Check sheet for the modelled part. Datum: model origin and axes. Units: mm. Give positions to 0.01 mm unless a question says otherwise; leave off trailing zeros. Write each loop counter-clockwise with the first axis right and the second up, starting at its lowest first coordinate (ties: lowest second). Pieces come first, ordered by that corner, then holes. Notation, with made-up numbers: M -7,53 L 3,53 A33 ccw 3,89 Z; hole C 44.25,-10.5 d5. An arc over 180 degrees is marked long. Write item = value, one per line. Start each with the question number.
1) Scan lines: line 1 along Z through (x, y) = (1, 7); line 2 along Z through (x, y) = (1.5, 67.5). Record each from-to range of solid material in increasing order. Write a range as [from, to].
2) Cross-section at A-A, the plane y = 38.5. Record the cut outline in (x, z), plus the area to 3 significant figures.
3) Go/stop test with a flat-tipped pin: pin 1 (1.5 mm diameter, centred on y = 38, z = 29.5, fed in from +X). Record where the tip stops, or that it passes through.
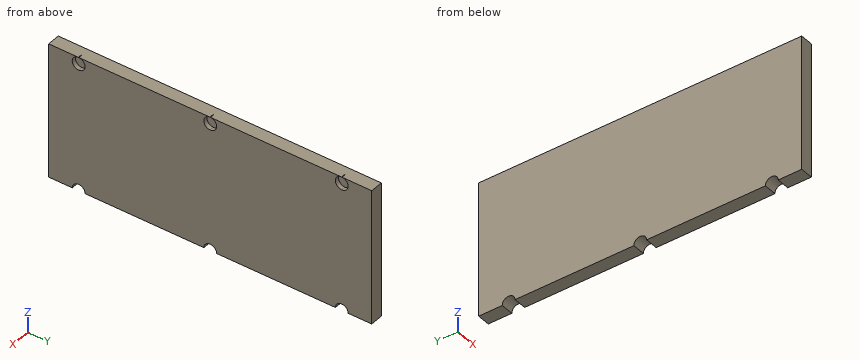
```python
from build123d import *

# Parameters (mm, degrees)
SKETCH_1_W                                     = 3
SKETCH_1_H                                     = 74
EXTRUDE_1_DEPTH                                = 31.5
SKETCH_2_W                                     = 3
SKETCH_2_H                                     = 1.5
SIDE_REAR_EXTENSION_1P5MM_DEPTH                = 31.5
SKETCH_3_R                                     = 1.5
SIDE_TOP_EDGE_MAGNET_POCKETS_D3_DEPTH1_3_DEPTH = 1
SIDE_BOTTOM_EDGE_SEMICIRCLES_D3_THROUGH_DEPTH  = 4


with BuildPart() as part:
    # Эскиз1 → Бобышка-Вытянуть1 (new body)
    with BuildSketch(Plane.XY):
        with Locations((1.5, 37)):
            Rectangle(SKETCH_1_W, SKETCH_1_H)
    extrude(amount=EXTRUDE_1_DEPTH)

    # Эскиз2 → side_rear_extension_1p5mm (add)
    with BuildSketch(Plane.XY):
        with Locations((1.5, 74.75)):
            Rectangle(SKETCH_2_W, SKETCH_2_H)
    extrude(amount=SIDE_REAR_EXTENSION_1P5MM_DEPTH)

    # Эскиз3 → side_top_edge_magnet_pockets_D3_depth1_3x (cut)
    with BuildSketch(Plane(origin=(3, 0, 0), x_dir=(0, 0, -1), z_dir=(1, 0, 0))):
        with Locations((-30.001, 7)):
            Circle(SKETCH_3_R)
        with Locations((-30.001, 37.75)):
            Circle(SKETCH_3_R)
        with Locations((-30.001, 68.5)):
            Circle(SKETCH_3_R)
    extrude(amount=-SIDE_TOP_EDGE_MAGNET_POCKETS_D3_DEPTH1_3_DEPTH, mode=Mode.SUBTRACT)

    # Эскиз4 → side_bottom_edge_semicircles_D3_through_3x (cut)
    with BuildSketch(Plane.ZY):
        with BuildLine():
            Line((0, 5.5), (0, 8.5))
            ThreePointArc((0, 8.5), (1.5, 7), (0, 5.5))
        make_face()
        with BuildLine():
            Line((0, 36.25), (0, 39.25))
            ThreePointArc((0, 39.25), (1.5, 37.75), (0, 36.25))
        make_face()
        with BuildLine():
            Line((0, 67), (0, 70))
            ThreePointArc((0, 70), (1.5, 68.5), (0, 67))
        make_face()
    extrude(amount=-SIDE_BOTTOM_EDGE_SEMICIRCLES_D3_THROUGH_DEPTH, mode=Mode.SUBTRACT)


solid = part.part
```
Reply:
q1.line_1 = [1.5, 31.5]
q1.line_2 = [1.12, 31.5]
q2.outline = M 0,1.3 L 3,1.3 L 3,28.7 L 2,28.7 L 2,31.3 L 3,31.3 L 3,31.5 L 0,31.5 Z
q2.area = 88.0 mm2
q3.pin_1 = 2
